Geometry: final body of the model. Coordinates: model frame, mm. A direction names the side the tool comes from. Give positions to 0.01 mm unless a question says otherwise; leave off trailing zeros. Loops run counter-clockwise (first coordinate to the right, second up) from the corner with the lowest first, then second, coordinate; pieces in that order, holes last. Notation, with made-up numbers: (38.25, -20.5) -> (78.25, -20.5) arc R20 cw to (78.25, 13.5) -> close; hole circle Ø3 at (4, 77). An arc over 180 degrees is marked (long way). One line per question, with ' | ' between items. Start each with the question number.
Item 1: Material intervals for line 1 along Z through (x, y) = (0, 1.3) (3 decimals); line 2 along Z through (x, y) = (111, 1.25); line 3 along Z through (x, y) = (74, 1.25), sorted ascending. Write a range as [from, to].
Item 2: Pin query (flat end, axial travel): P1, Ø1.5, axis at y = 0.5, z = 75.5, coming from the -X side; P2, Ø1.7, axis at x = 76, y = 2.5, coming from the +Z side; P3, Ø0.9, axis at x = 101, y = 1, coming from the -Z side. Return the tip coordinate at first contact, or that it passes through.
Item 3: Section D-D on x = 67.5. Return loops of the section in (y, z).
Item 4: Section C-C on z = 71. Return loops of the section in (x, y), then the cut area to 3 significant figures.
Item 5: Mould query, pull axis X, two halves, no side actions, for faces 1 (the flat face through (88, 1.524, 99)), 2 (the flat face through (91.65, 0.75, 116.02)), 3 (the flat face through (104.266, 0.751, 109.563)). Classes: released by +X, released by -X, zero draft, split by the parting line, or undercut.
Item 6: Section A-A on x = 130.5. Return loops of the section in (y, z), then the cut area to 3 significant figures.
Item 7: Set-up query: faces 4 (the flat face through (72.45, 0.75, 109.56)), 5 (the flat face through (85.062, 0.751, 116.021)), 6 (the cylindrical face through (192.583, 1.503, -0.626)). Return all of +Z, -Z, +X, -X, +Y, -Y with unobstructed straight access to the full face (end or side cutting, diameter ignored); none if empty.
Item 8: Section B-B on y = 2. Give the number of separate pieces and of enclosed holes in the cut face, then the cut area to 3 significant figures.
Autodesk Inventor part; units mm, degrees
ref_plane "Work Plane1" through (15.0403, 0, 98.425) normal (0, 0, 1) x (1, 0, 0)
ref_plane "YZ Plane" through (0, 0, 0) normal (1, 0, 0) x (0, 1, 0)
ref_plane "XZ Plane" through (0, 0, 0) normal (0, 1, 0) x (-1, 0, 0)
sketch "Sketch1" plane through (0, 0, 0) normal (0, 1, 0) x (-1, 0, 0)
  circle A0 centre (0, 0) radius 3.175
  circle A1 centre (0, -9.6012) radius 1.5875
  circle A2 centre (8.1026, 0) radius 1.5875
  circle A3 centre (0, 9.6012) radius 1.5875
  circle A4 centre (-8.1026, 0) radius 1.5875
  circle A5 centre (0, 0) radius 15.875
  circle A6 centre (-176.7205, 0) radius 3.175
  circle A7 centre (-176.7332, -9.6012) radius 1.5875
  circle A8 centre (-184.8358, 0) radius 1.5875
  circle A9 centre (-176.7332, 9.6012) radius 1.5875
  circle A10 centre (-168.6306, 0) radius 1.5875
  circle A11 centre (-176.7205, 0) radius 15.875
  line L0 (-163.5506, 5.08) -> (-13.1826, 5.08)
  line L1 (-13.1826, 5.08) -> (-13.1826, -5.08)
  line L2 (-13.1826, -5.08) -> (-163.5506, -5.08)
  line L3 (-163.5506, -5.08) -> (-163.5506, 5.08)
  line L4 (0, 0) -> (-163.5506, 0)
  line L5 (-170.2181, 0) -> (-176.7078, 0)
  line L6 (-176.7205, 0) -> (-170.2181, 0)
  line L7 (-167.0431, 0) -> (-0.0127, 0)
  line L8 (-176.7078, 0) -> (-170.2181, 0)
  line L9 (-167.0431, 0) -> (-88.3666, 0)
  point P0 (-161.6802, -5.08)
  point P1 (-15.0403, -5.08)
  point P2 (-15.0403, 5.08)
  point P3 (-161.6802, 5.08)
  dimension "d0" = 6.35
  dimension "d1" = 3.175
  dimension "d2" = 3.175
  dimension "d3" = 3.175
  dimension "d4" = 3.175
  dimension "d5" = 9.6012
  dimension "d6" = 8.1026
  dimension "d7" = 8.1026
  dimension "d8" = 9.6012
  dimension "d9" = 31.75
  dimension "d14" = 5.08
  dimension "d15" = 5.08
  dimension "d16" = 5.08
  dimension "d17" = 5.08
  dimension "d50" = 176.7078
extrude "Extrusion1" add sketch "Sketch1" along normal blind 3.048
ref_plane "Work Plane1" through (15.0403, 0, 98.425) normal (0, 0, 1) x (1, 0, 0)
mirror "Mirror1" [suppressed]
sketch "Sketch2" plane through (0, 3.048, 0) normal (0, 1, 0) x (1, 0, 0)
  arc A0 (15.0403, 5.08) -> (15.0403, -5.08) centre (0, 0) ccw
  line L0 (158.3147, -191.0461) -> (27.7403, 5.8039)
  arc A1 (161.6802, -5.08) -> (161.6802, 5.08) centre (176.7205, 0) ccw
  line L1 (18.143, -191.4206) -> (148.9802, 5.8039)
  line L2 (17.5803, -4.3561) -> (147.9282, -200.8645)
  line L3 (161.6802, -5.08) -> (159.1402, -5.08)
  line L4 (159.1402, -4.3561) -> (28.303, -201.5806)
  line L5 (95.3776, -74.9969) -> (112.2777, -74.9969)
  line L6 (81.337, -74.9969) -> (64.4377, -74.9969)
  line L7 (95.0379, -75.509) -> (111.9379, -75.509)
  line L8 (81.6767, -75.509) -> (64.7774, -75.509)
  line L9 (96.8065, -99.0548) -> (79.9064, -99.0548)
  line L10 (88.3569, -86.3038) -> (88.3569, -85.5799)
  line L11 (161.6802, 5.08) -> (15.0403, 5.08)
  line L12 (88.3569, -86.3038) -> (89.0808, -86.3038) construction
  line L13 (81.1864, -121.864) -> (64.2863, -121.864)
  line L14 (95.5256, -121.864) -> (112.4249, -121.864)
  line L15 (15.0403, -5.08) -> (161.6802, -5.08)
  line L16 (34.9598, -5.08) -> (18.0604, -5.08)
  line L17 (141.7599, -5.08) -> (159.1402, -5.08)
  point P0 (79.9068, -98.3176)
  point P1 (88.3564, -111.0559)
  point P2 (96.8065, -98.3182)
  point P3 (88.3569, -85.5799)
  point P4 (64.5631, -75.9099)
  point P5 (81.4625, -75.9099)
  point P6 (95.0379, -75.509)
  point P7 (158.66, -5.08)
  point P8 (141.7599, -5.08)
  dimension "d69" = 23.5458
  dimension "d70" = 23.5458
  dimension "d81" = 90
  dimension "d82" = 22.8092
  dimension "d83" = 22.8092
extrude "Extrusion2" add sketch "Sketch2" against normal blind 3.048 contours L15 L0 L6 L2 | L6 L0 L8 L2 | L15 L4 L5 L1 | L5 L4 L7 L1
sketch "Sketch3" plane through (0, 0, 0) normal (0, -1, 0) x (1, 0, 0)
  line L0 (34.9598, 5.08) -> (81.6767, 75.509)
  line L1 (64.7774, 75.509) -> (18.0604, 5.08)
  line L2 (18.0604, 5.08) -> (159.8416, 218.8249)
  line L3 (15.0403, 5.08) -> (161.6802, 5.08)
  line L4 (34.9598, 5.08) -> (173.1628, 213.4305)
  line L5 (15.0403, 5.08) -> (161.6802, 5.08)
  line L6 (158.66, 5.08) -> (122.9182, 58.9573)
  line L7 (158.66, 5.08) -> (111.9379, 75.509)
  line L8 (158.66, 5.08) -> (25.1448, 206.3412)
  line L9 (141.7599, 5.08) -> (8.7682, 205.5521)
  line L10 (95.3776, 74.9969) -> (112.2777, 74.9969)
  line L11 (112.162, 75.4579) -> (95.2201, 75.4579)
  line L12 (64.4377, 74.9969) -> (81.337, 74.9969)
  line L13 (81.337, 75.7208) -> (64.4377, 75.7208)
  line L14 (81.675, 121.1274) -> (64.775, 121.1274)
  line L15 (111.9363, 121.1274) -> (95.037, 121.1274)
  line L16 (64.7774, 75.509) -> (81.6767, 75.509)
  line L17 (95.1415, 75.3529) -> (112.0415, 75.3529)
  line L18 (79.9064, 98.3182) -> (96.8065, 98.3182)
  point P0 (0, 0)
  point P1 (18.0604, 5.08)
  point P2 (141.7599, 5.08)
  point P3 (173.1628, 213.4305)
  point P4 (8.7682, 205.5521)
  point P5 (81.337, 74.9969)
  point P6 (88.3569, 85.5799)
  point P7 (112.2777, 74.9969)
  point P8 (96.6135, 98.7512)
  point P9 (88.3564, 111.0559)
  point P10 (79.9068, 98.3176)
  point P11 (95.3776, 74.9969)
  point P12 (81.4625, 75.9099)
  point P13 (64.5631, 75.9099)
  point P14 (111.9379, 75.509)
  dimension "d58" = 22.8092
  dimension "d64" = 22.8092
  dimension "d65" = 22.8092
  dimension "d67" = 22.9653
extrude "Extrusion3" add sketch "Sketch3" against normal blind 1.524 contours L16 L2 L9 L4 | L9 L18 L4 | L4 L8 L7 L17 L9 | L8 L2 L15 L4 | L18 L2 L8 | L9 L14 L8 L2
sketch "Sketch4" plane through (0, 1.524, 0) normal (0, 1, 0) x (1, 0, 0)
  line L0 (111.9363, -121.1274) -> (96.8065, -98.3182)
  line L1 (79.9068, -98.3176) -> (64.775, -121.1274)
  line L2 (158.66, -5.08) -> (96.8065, -98.3182)
  line L3 (88.3564, -111.0559) -> (95.037, -121.1274)
  line L4 (96.8065, -98.3182) -> (88.3564, -111.0559)
  line L5 (96.8065, -98.3182) -> (88.3569, -85.5799)
  line L6 (88.3569, -85.5799) -> (88.3564, -111.0559)
  line L7 (79.9068, -98.3176) -> (88.3564, -111.0559)
  line L8 (96.8065, -98.3182) -> (79.9068, -98.3176)
  line L9 (88.3566, -98.3179) -> (78.3429, -83.2215)
  line L10 (88.3569, -85.5799) -> (96.8065, -98.3182)
  line L11 (88.3566, -98.3179) -> (98.3715, -83.2215)
  line L12 (95.0379, -75.509) -> (88.3569, -85.5799)
  line L13 (78.3429, -83.2215) -> (98.3715, -83.2215)
  line L14 (78.3429, -83.2215) -> (96.1304, -110.0373)
  line L15 (98.3715, -83.2215) -> (80.5501, -110.0856)
  circle A0 centre (88.3566, -98.3179) radius 18.1163
  line L16 (88.3566, -98.3179) -> (98.3708, -113.4149)
  line L17 (88.3566, -98.3179) -> (78.3425, -113.4149)
  circle A1 centre (78.3429, -83.2215) radius 1.5875
  circle A2 centre (98.3715, -83.2215) radius 1.5875
  circle A3 centre (98.3708, -113.4149) radius 1.5875
  circle A4 centre (78.3425, -113.4149) radius 1.5875
  point P0 (0, 0)
  point P1 (87.8755, -85.578)
  point P2 (87.8599, -111.6467)
  point P3 (111.9412, -75.1032)
  point P4 (64.2633, -75.4579)
  point P5 (112.162, -75.4579)
  point P6 (34.9598, -5.08)
  point P7 (18.0604, -5.08)
  point P8 (81.1626, -75.4579)
  point P9 (95.2356, -75.4579)
  point P10 (95.1415, -76.0768)
  point P11 (81.6767, -76.2329)
  point P12 (64.5631, -75.9099)
  point P13 (64.7549, -76.199)
  point P14 (112.2777, -74.9969)
  dimension "d74" = 3.175
  dimension "d75" = 3.175
  dimension "d76" = 3.175
  dimension "d77" = 3.175
  dimension "d78" = 33.559
  dimension "d79" = 33.558
extrude "Extrusion4" cut sketch "Sketch4" against normal blind 3.81 contours A3 A0 | A0 L16 A3 | A0 A3 L16 | A2 L11 A0 | A0 A2 | A2 L13 L11 | A1 A0 L9 | L9 L13 A1 | L13 A2 A0 | A0 A1 L13 | A0 A1 | A4 A0 | A0 L17 A4 | A4 L17 A0
properties part number "crossBraces"
Result sheet:
1) line 1: z = [-15.875, -11.189], [-8.014, -3.175], [3.175, 8.014], [11.189, 15.875] | line 2: z = [-5.08, 5.08], [51.45, 76.92], [119.72, 121.13] | line 3: z = [-5.08, 5.08], [63.94, 89.41], [107.22, 121.13]
2) P1: stops at x = 64.27 | P2: stops at z = 75.51 | P3: stops at z = -5.08
3) outline: (0, -5.08) -> (3.05, -5.08) -> (3.05, 5.08) -> (0, 5.08) -> close; (0, 54.14) -> (3.05, 54.14) -> (3.05, 75.51) -> (1.52, 75.51) -> (1.52, 79.61) -> (0, 79.61) -> close; (0, 117.02) -> (1.52, 117.02) -> (1.52, 121.13) -> (0, 121.13) -> close
4) outline: (61.79, 0) -> (78.69, 0) -> (78.69, 3.05) -> (61.79, 3.05) -> close; (98.03, 0) -> (114.93, 0) -> (114.93, 3.05) -> (98.03, 3.05) -> close | area: 103 mm²
5) face 1: zero draft | face 2: undercut | face 3: released by +X
6) outline: (0, -5.08) -> (3.05, -5.08) -> (3.05, 5.08) -> (0, 5.08) -> close; (0, 22.05) -> (3.05, 22.05) -> (3.05, 47.53) -> (0, 47.53) -> close | area: 109 mm²
7) face 4: -X, +Y, -Y | face 5: +Z, +Y, -Y | face 6: +Y, -Y
8) separate pieces: 1 | enclosed holes: 10 | area: 5,320 mm²
